```python
from build123d import *

# Parameters (mm, degrees)
CROQUIS1_R              = 5
CROQUIS1_R_2            = 1.5
SALIENTE_EXTRUIR1_DEPTH = 2
CHAFL_N1_SIZE           = 1


with BuildPart() as part:
    # Croquis1 → Saliente-Extruir1 (new body)
    with BuildSketch(Plane.XY):
        with BuildLine():
            Line((-67.5, -20.5), (67.5, -20.5))
            ThreePointArc((67.5, -20.5), (71.035533906, -19.035533906), (72.5, -15.5))
            Line((72.5, -15.5), (72.5, 15.5))
            ThreePointArc((72.5, 15.5), (71.035533906, 19.035533906), (67.5, 20.5))
            Line((67.5, 20.5), (-67.5, 20.5))
            ThreePointArc((-67.5, 20.5), (-71.035533906, 19.035533906), (-72.5, 15.5))
            Line((-72.5, 15.5), (-72.5, -15.5))
            ThreePointArc((-72.5, -15.5), (-71.035533906, -19.035533906), (-67.5, -20.5))
        make_face()
        with Locations((-52.5, -1.5)):
            Circle(CROQUIS1_R, mode=Mode.SUBTRACT)
        with Locations((-17.5, -1.5)):
            Circle(CROQUIS1_R, mode=Mode.SUBTRACT)
        with Locations((17.5, -1.5)):
            Circle(CROQUIS1_R, mode=Mode.SUBTRACT)
        with Locations((52.5, -1.5)):
            Circle(CROQUIS1_R, mode=Mode.SUBTRACT)
        with Locations((-66, 14)):
            Circle(CROQUIS1_R_2, mode=Mode.SUBTRACT)
        with Locations((-66, -14)):
            Circle(CROQUIS1_R_2, mode=Mode.SUBTRACT)
        with Locations((66, -14)):
            Circle(CROQUIS1_R_2, mode=Mode.SUBTRACT)
        with Locations((66, 14)):
            Circle(CROQUIS1_R_2, mode=Mode.SUBTRACT)
    extrude(amount=-SALIENTE_EXTRUIR1_DEPTH)

    # Chaflán1
    chafl_n1_edges = [part.edges().sort_by_distance(p)[0] for p in [
        (-67.5, 14, 0),
        (-67.5, -14, 0),
        (64.5, -14, 0),
        (64.5, 14, 0),
    ]]
    chamfer(chafl_n1_edges, length=CHAFL_N1_SIZE)


solid = part.part
```
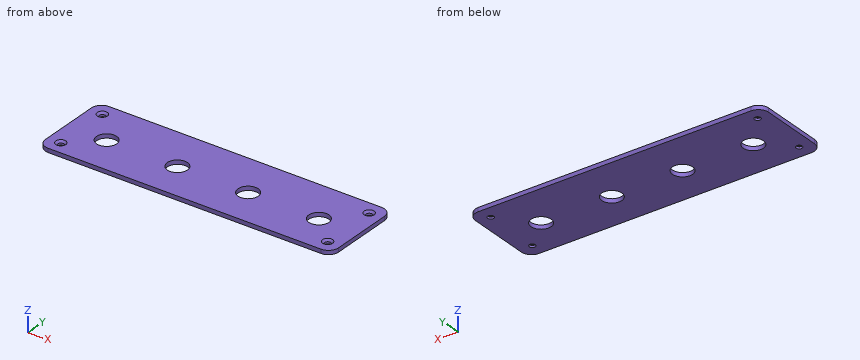
The model under review builds one solid part; all positions refer to its coordinate system, in mm. Round coordinates to 2 decimals unless told otherwise and drop trailing zeros. Order: outer loops, then holes, each group sorted by start corner. A loop starts at its lowest first (then second) coordinate and runs counter-clockwise, first axis right, second up. Notation, with made-up numbers: (11, 18.5) -> (30, 18.5) arc R12 cw to (30, 28.5) -> close; hole circle Ø3 at (76.25, -20.75). An arc over 180 degrees is marked (long way). One line per item, written item: value. Start each with the question number.
Q1. Take a section at B-B (y = 1). Write out the cut boundary in (x, z), and give its area (3 significant figures).
Q2. Take a section at A-A (x = -17.5). Write out the cut boundary in (y, z), and give its area (3 significant figures).
Q3. Wall thickness on line 1 (Y direction, x = -66, z = -1.5); line 2 (X direction, y = 3, z = -0.65); line 3 (X direction, y = -13, z = -0.9): over which ranges is each line inside the solid? List them lowest first.
Q4. Clearance check with a flat-ended pin moving along its axis: pin 1 Ø6 at (x, y) = (-17.5, -1.5) entering from -Z. State where the tip first meets the part, or that it passes through.
Q5. Take a section at C-C (x = -66). Write out the cut boundary in (y, z).
Reported:
1. outline: (-72.5, -2) -> (-56.83, -2) -> (-56.83, 0) -> (-72.5, 0) -> close; (-48.17, -2) -> (-21.83, -2) -> (-21.83, 0) -> (-48.17, 0) -> close; (-13.17, -2) -> (13.17, -2) -> (13.17, 0) -> (-13.17, 0) -> close; (21.83, -2) -> (48.17, -2) -> (48.17, 0) -> (21.83, 0) -> close; (56.83, -2) -> (72.5, -2) -> (72.5, 0) -> (56.83, 0) -> close
1. area: 221 mm2
2. outline: (-20.5, -2) -> (-6.5, -2) -> (-6.5, 0) -> (-20.5, 0) -> close; (3.5, -2) -> (20.5, -2) -> (20.5, 0) -> (3.5, 0) -> close
2. area: 62.0 mm2
3. line 1: y = -20.5 to -15.5, -12.5 to 12.5, 15.5 to 20.5
3. line 2: x = -72.5 to -54.68, -50.32 to -19.68, -15.32 to 15.32, 19.68 to 50.32, 54.68 to 72.5
3. line 3: x = -72.5 to -67.25, -64.75 to 64.75, 67.25 to 72.5
4. pin 1: passes through
5. outline: (-20.5, -2) -> (-15.5, -2) -> (-15.5, -1) -> (-16.5, 0) -> (-20.5, 0) -> close; (-12.5, -2) -> (12.5, -2) -> (12.5, -1) -> (11.5, 0) -> (-11.5, 0) -> (-12.5, -1) -> close; (15.5, -2) -> (20.5, -2) -> (20.5, 0) -> (16.5, 0) -> (15.5, -1) -> close
